Check sheet for the modelled part. Datum: model origin and axes. Units: mm. Give positions to 0.01 mm unless a question says otherwise; leave off trailing zeros. Write each loop counter-clockwise with the first axis right and the second up, starting at its lowest first coordinate (ties: lowest second). Pieces come first, ordered by that corner, then holes. Notation, with made-up numbers: M 36,31 L 47,31 A6 cw 47,40 Z; hole C -4,57.5 d6. An arc over 180 degrees is marked long. Write item = value, one per line. Start each with the question number.
1) Scan lines: L1, parallel to Z at x = 0, y = 3; L2, parallel to X at y = 4.75, z = 77. Record each from-to range of solid material in increasing order.
2) Gauge pin test, flat end, axial feed: pin 1 (6 mm diameter, centred on x = 76.01, z = -76.01, fed in from -Y). Record the tip position at first contact, or that the pin passes through.
3) Sectioned sample at A-A, the plane z = 0. Record the cut outline in (x, y).
4) Sectioned sample at C-C, the plane y = 3.75. Record the cut outline in (x, z).
5) Sectioned sample at B-B, the plane x = -18.5. Record the cut outline in (y, z).
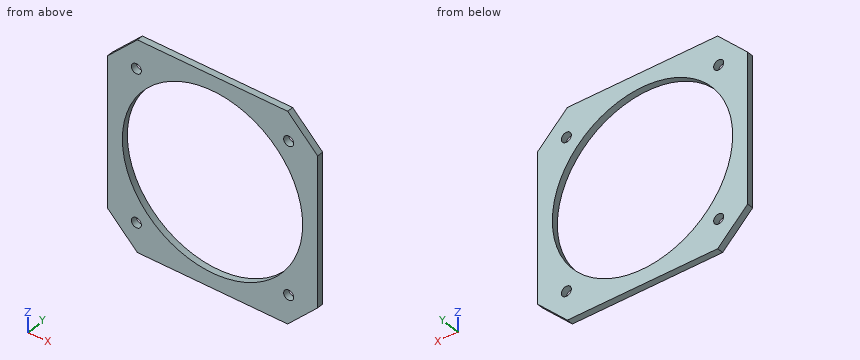
from build123d import *

# Parameters (mm, degrees)
SKETCH1_W           = 210
SKETCH1_H           = 210
SKETCH1_R           = 90
SKETCH1_R_2         = 5
BOSS_EXTRUDE1_DEPTH = 6.35
CHAMFER1_SIZE       = 30


with BuildPart() as part:
    # Sketch1 → Boss-Extrude1 (new body)
    with BuildSketch(Plane(origin=(0, 0, 0), x_dir=(1, 0, 0), z_dir=(0, 1, 0))):
        Rectangle(SKETCH1_W, SKETCH1_H)
        Circle(SKETCH1_R, mode=Mode.SUBTRACT)
        with Locations((-76.013978978, 76.013978978)):
            Circle(SKETCH1_R_2, mode=Mode.SUBTRACT)
        with Locations((76.013978978, 76.013978978)):
            Circle(SKETCH1_R_2, mode=Mode.SUBTRACT)
        with Locations((76.013978978, -76.013978978)):
            Circle(SKETCH1_R_2, mode=Mode.SUBTRACT)
        with Locations((-76.013978978, -76.013978978)):
            Circle(SKETCH1_R_2, mode=Mode.SUBTRACT)
    extrude(amount=BOSS_EXTRUDE1_DEPTH)

    # Chamfer1
    chamfer1_edges = [part.edges().sort_by_distance(p)[0] for p in [
        (105, 3.175, 105),
        (-105, 3.175, 105),
        (-105, 3.175, -105),
        (105, 3.175, -105),
    ]]
    chamfer(chamfer1_edges, length=CHAMFER1_SIZE)


solid = part.part
Data:
q1.L1 = -105 to -90, 90 to 105
q1.L2 = -103 to -80.92, -71.11 to -46.59, 46.59 to 71.11, 80.92 to 103
q2.pin_1 = through
q3.outline = M -105,0 L -90,0 L -90,6.35 L -105,6.35 Z; M 90,0 L 105,0 L 105,6.35 L 90,6.35 Z
q4.outline = M -105,-75 L -75,-105 L 75,-105 L 105,-75 L 105,75 L 75,105 L -75,105 L -105,75 Z; hole C 0,0 d180; hole C -76.01,-76.01 d10; hole C -76.01,76.01 d10; hole C 76.01,-76.01 d10; hole C 76.01,76.01 d10
q5.outline = M 0,-105 L 6.35,-105 L 6.35,-88.08 L 0,-88.08 Z; M 0,88.08 L 6.35,88.08 L 6.35,105 L 0,105 Z
